Verification items for the finished model (mm, model axes). Give positions to 0.01 mm unless a question says otherwise; leave off trailing zeros. Order: outer loops, then holes, each group sorted by start corner. A loop starts at its lowest first (then second) coordinate and runs counter-clockwise, first axis right, second up.
(1) Sectioned sample at D-D on z = -26.5. Record the cut outline in (x, y).
(2) Sectioned sample at C-C on y = 85. Record the cut outline in (x, z), plus the area to 3 significant figures.
(3) Gauge pin test, flat end, axial feed: pin 1 (6 mm diameter, centred on x = 6.5, z = -2.5, fed in from -Y). Record the tip position at first contact, or that the pin passes through.
(4) Sectioned sample at B-B on x = 10. Record the cut outline in (y, z), plus the area to 3 significant figures.
(5) Scan lines: L1, parallel to Z at x = 9, y = 85; L2, parallel to Z at x = 23, y = 80; L3, parallel to Y at x = 18.5, z = -6.5. Record each from-to range of solid material in increasing order.
(6) Sectioned sample at A-A on z = 0. Record the cut outline in (x, y), plus the area to 3 significant figures.
(7) Mould release check, pull along Z, two halves, no side actions. Record for faces 1 (the face through (12, -2, 31.5)), 2 (the face through (25, 2, 0)), 3 (the face through (12.325, -103.832, -0.477)): pulls with the +Z half, pulls with the -Z half, needs draft (parallel to the pull), parting line crosses it, or undercut.
```python
from build123d import *

# Parameters (mm, degrees)
BOSS_EXTRUDE1_DEPTH     = 25
CUT_EXTRUDE1_DEPTH      = 122.828773284
CUT_EXTRUDE1_DEPTH_BACK = 122.828773284
SKETCH2_R               = 18.5


with BuildPart() as part:
    # Sketch1 → Boss-Extrude1 (new body)
    with BuildSketch(Plane(origin=(0, 0, 0), x_dir=(0, 0, -1), z_dir=(1, 0, 0))):
        with BuildLine():
            Line((-31.5, -115), (-31.5, 115))
            Line((-31.5, 115), (31.5, 115))
            Line((31.5, 115), (31.5, -115))
            ThreePointArc((31.5, -115), (0, -103.829756631), (-31.5, -115))
        make_face()
    extrude(amount=BOSS_EXTRUDE1_DEPTH)

    # Sketch2 → Cut-Extrude1 (cut, two sides: drawn at the far end of the back side and taken through both)
    with BuildSketch(Plane(origin=(25, 0, 0), x_dir=(0, 0, -1), z_dir=(1, 0, 0)).offset(-CUT_EXTRUDE1_DEPTH_BACK)):
        with Locations((0, 85)):
            Circle(SKETCH2_R)
    extrude(amount=CUT_EXTRUDE1_DEPTH + CUT_EXTRUDE1_DEPTH_BACK, mode=Mode.SUBTRACT)


solid = part.part
```
Ans:
1. outline: (0, -111.43) - (25, -111.43) - (25, 115) - (0, 115) - close
2. outline: (0, -31.5) - (25, -31.5) - (25, -18.5) - (0, -18.5) - close; (0, 18.5) - (25, 18.5) - (25, 31.5) - (0, 31.5) - close
2. area: 650 mm2
3. pin 1: stops at y = -104.13
4. outline: (-115, -31.5) - (115, -31.5) - (115, 31.5) - (-115, 31.5) arc R50 cw to start; hole circle Ø37 at (85, 0)
4. area: 12,900 mm2
5. L1: z = -31.5 to -18.5, 18.5 to 31.5
5. L2: z = -31.5 to -17.81, 17.81 to 31.5
5. L3: y = -104.25 to 67.68, 102.32 to 115
6. outline: (0, -103.83) - (25, -103.83) - (25, 66.5) - (0, 66.5) - close; (0, 103.5) - (25, 103.5) - (25, 115) - (0, 115) - close
6. area: 4,550 mm2
7. face 1: pulls with the +Z half
7. face 2: needs draft
7. face 3: undercut
